```python
from build123d import *

# Parameters (mm, degrees)
F1_DEPTH = 50
F2_R     = 11.5
F3_DEPTH = 64
F4_R     = 14
F5_DEPTH = 62
F6_R     = 9.504259
F6_R_2   = 9.5
F7_DEPTH = 58
F8_R     = 17
F9_DEPTH = 23


with BuildPart() as f1:
    # F0 (on Front) → F1 (new body)
    with BuildSketch(Plane.XZ):
        with BuildLine():
            ThreePointArc((-106.73253, 26.611409), (-79.062913, 76.47912), (-30.141732, 105.789773))
            ThreePointArc((-30.141732, 105.789773), (0, 123), (30.141732, 105.789773))
            ThreePointArc((30.141732, 105.789773), (79.062913, 76.47912), (106.73253, 26.611409))
            Line((106.73253, 26.611409), (115.068493, -6.822315))
            ThreePointArc((115.068493, -6.822315), (112.580369, -45.473999), (92.227353, -78.426968))
            ThreePointArc((92.227353, -78.426968), (92.277337, -101.381582), (115.220751, -100.66285))
            ThreePointArc((115.220751, -100.66285), (128.638477, -91.018209), (144.809642, -87.619991))
            ThreePointArc((144.809642, -87.619991), (165.992581, -71.632085), (156.379154, -46.895229))
            ThreePointArc((156.379154, -46.895229), (145.085673, -36.45592), (138.565787, -22.527067))
            Line((138.565787, -22.527067), (125.168149, 31.207925))
            ThreePointArc((125.168149, 31.207925), (108.494033, 69.785707), (80.304388, 100.956452))
            Line((80.304388, 100.956452), (36.575319, 135.740125))
            ThreePointArc((36.575319, 135.740125), (26.653961, 147.361151), (21.814031, 161.854483))
            ThreePointArc((21.814031, 161.854483), (3.277246, 180.754532), (-20.004938, 168.154367))
            ThreePointArc((-20.004938, 168.154367), (-28.641021, 157.133884), (-41.3379, 151.232848))
            ThreePointArc((-41.3379, 151.232848), (-50.681665, 146.131487), (-55.509144, 136.643322))
            ThreePointArc((-55.509144, 136.643322), (-62.367303, 118.652566), (-75.515118, 104.587126))
            ThreePointArc((-75.515118, 104.587126), (-106.838992, 72.294051), (-125.168149, 31.207925))
            Line((-125.168149, 31.207925), (-138.565787, -22.527067))
            ThreePointArc((-138.565787, -22.527067), (-145.085673, -36.45592), (-156.379154, -46.895229))
            ThreePointArc((-156.379154, -46.895229), (-165.992581, -71.632085), (-144.809642, -87.619991))
            ThreePointArc((-144.809642, -87.619991), (-128.638477, -91.018209), (-115.220751, -100.66285))
            ThreePointArc((-115.220751, -100.66285), (-92.277337, -101.381582), (-92.227353, -78.426968))
            ThreePointArc((-92.227353, -78.426968), (-112.580369, -45.473999), (-115.068493, -6.822315))
            Line((-115.068493, -6.822315), (-106.73253, 26.611409))
        make_face()
    extrude(amount=-F1_DEPTH)

    # F2 (on Front) → F3 (cut)
    with BuildSketch(Plane.XZ):
        with Locations((0, 159)):
            Circle(F2_R)
        with Locations((144.83, -65.62)):
            Circle(F2_R)
        with Locations((-144.83, -65.62)):
            Circle(F2_R)
    extrude(amount=-F3_DEPTH, mode=Mode.SUBTRACT)

    # F4 (on Front) → F5 (cut)
    with BuildSketch(Plane.XZ):
        with Locations((-37.77, 127.52)):
            Circle(F4_R)
    extrude(amount=-F5_DEPTH, mode=Mode.SUBTRACT)

    # F6 (on Front) → F7 (cut)
    with BuildSketch(Plane.XZ):
        with Locations((-103.4, -89.88)):
            Circle(F6_R)
        with Locations((103.4, -89.88)):
            Circle(F6_R_2)
    extrude(amount=-F7_DEPTH, mode=Mode.SUBTRACT)

    # F8 (on face) → F9 (cut)
    with BuildSketch(Plane(origin=(0, 50, 0), x_dir=(-1, 0, 0), z_dir=(0, 1, 0))):
        with Locations((-144.83, -65.62)):
            Circle(F8_R)
        with Locations((144.83, -65.62)):
            Circle(F8_R)
        with Locations((0, 159)):
            Circle(F8_R)
    extrude(amount=-F9_DEPTH, mode=Mode.SUBTRACT)


solid = f1.part
```
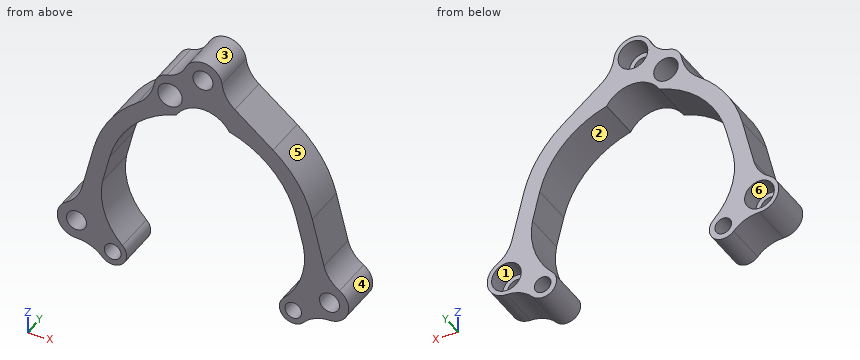
Source: CAD feature listing. Evaluate the final solid. Frame: model axes, mm. Face numbers are marked on the shaded views. A direction names the side the tool comes from. Coordinates: 2 decimals unless noted, no trailing zeros. Order: outer loops, then holes, each group sorted by start corner. A loop starts at its lowest first (then second) coordinate and runs counter-clockwise, first axis right, second up. Notation, with made-up numbers: M 22.5,54.25 L 57.5,54.25 A34 cw 57.5,90.25 Z; hole C 14,54 d9. An arc over 180 degrees is marked long. Write each question's results on one line, items separated by ' | '. Start each with the question number.
1) Line query: line 1 (X direction, y = 5, z = -83.5); line 2 (X direction, y = 8, z = -67.5); line 3 (Z direction, x = 0, y = 42.25). Output: solid intervals per line, ascending. Write a range as from..to.
2) Section query B-B (x = 0). Return the cut outline in (y, z), plus the area to 3 significant figures.
3) Section query C-C (z = 42.5). Return the cut outline in (x, y), plus the area to 3 significant figures.
4) Access query for the marked faces 1, 2 and 3. Directions: +Z, -Z, +X, -X, +Y, -Y. A direction counts if a zero-diameter tool reaches every point of the face in a straight line with its end or side. Return the directions, or none.
5) Section query D-D (z = -65.62). Return the cut outline in (x, y).
6) Draft query along Z for the marked faces 4, 5 and 6. Return one class per face: released by +Z, released by -Z, zero draft, split by the parting line, or undercut.
7) Section query A-A (y = 33). Give the number of separate pieces and of enclosed holes in the cut face, plus the area to 3 significant figures.
8) Contact query for flat-ended pins moving along their axis: pin 1 Ø12 at (x, y) = (61, 6) entering from -Z; pin 2 Ø8 at (y, z) = (10.5, 71.5) entering from +X; pin 3 Ø5 at (y, z) = (20, 78.5) entering from +X. Output: stop coordinate, or through.
Answers:
1) line 1: x = -157.65..-110.44, -96.36..-88.73, 88.73..96.36, 110.44..157.65 | line 2: x = -166.75..-156.18, -133.48..-101.58, 101.58..133.48, 156.18..166.75 | line 3: z = 123..142, 176..181
2) outline: M 0,123 L 50,123 L 50,142 L 27,142 L 27,147.5 L 0,147.5 Z; M 0,170.5 L 27,170.5 L 27,176 L 50,176 L 50,181 L 0,181 Z | area: 1,500 mm^2
3) outline: M -121.8,0 L -101.46,0 L -101.46,50 L -121.8,50 Z; M 101.46,0 L 121.8,0 L 121.8,50 L 101.46,50 Z | area: 2,030 mm^2
4) face 1: +Y | face 2: +Y, -Y | face 3: +Z, +Y, -Y
5) outline: M -166.83,0 L -156.33,0 L -156.33,27 L -161.83,27 L -161.83,50 L -166.83,50 Z; M -133.33,0 L -102.87,0 L -102.87,50 L -127.83,50 L -127.83,27 L -133.33,27 Z; M 102.87,0 L 133.33,0 L 133.33,27 L 127.83,27 L 127.83,50 L 102.87,50 Z; M 156.33,0 L 166.83,0 L 166.83,50 L 161.83,50 L 161.83,27 L 156.33,27 Z
6) face 4: split by the parting line | face 5: released by +Z | face 6: undercut
7) separate pieces: 1 | enclosed holes: 6 | area: 14,900 mm^2
8) pin 1: stops at z = 87.24 | pin 2: stops at x = 109.93 | pin 3: stops at x = 104.24
